Geometry: final body of the model. Coordinates: model frame, mm. Round coordinates to 2 decimals unless told otherwise and drop trailing zeros. Loops run counter-clockwise (first coordinate to the right, second up) from the corner with the lowest first, then second, coordinate; pieces in that order, holes last. Notation, with made-up numbers: (-17.5, -32.5) - (11.5, -32.5) arc R25 ccw to (11.5, -17.5) - close; hole circle Ø9 at (-40, -2.75). An arc over 180 degrees is marked (long way). Answer as a JSON object with one key per item and string values. Group by question number.
Item 1: Line query: line 1 (Y direction, x = 10.75, z = 183); line 2 (X direction, y = 27.25, z = 531.5); line 3 (X direction, y = 22.25, z = 193). Output: solid intervals per line, ascending.
Item 2: Section A-A (z = 459). Return the cut outline in (x, y).
Item 3: Section B-B (y = 22). Return the cut outline in (x, z).
Item 4: First-contact query: pin 1 (10 mm diameter, centred on x = 12, z = 390, fed in from +Y); pin 2 (3 mm diameter, centred on y = 6.5, z = 320, fed in from -X); pin 3 (1.5 mm diameter, centred on x = -2, z = 293.5, fed in from +Y). Flat tips, straight axial feed; report the tip coordinate or a pass-through.
```python
from build123d import *

# Parameters (mm, degrees)
BOSS_EXTRUDE1_DEPTH = 600


with BuildPart() as part:
    # Sketch1 → Boss-Extrude1 (new body)
    with BuildSketch(Plane.XY):
        with BuildLine():
            Line((15, 0), (-15, 0))
            Line((-15, 0), (-15, 4.7625))
            Line((-15, 4.7625), (-6, 4.7625))
            Line((-6, 4.7625), (-6, 11.1125))
            Line((-6, 11.1125), (-2.783018763, 16.684474949))
            ThreePointArc((-2.783018763, 16.684474949), (0, 28), (2.783018763, 16.684474949))
            Line((2.783018763, 16.684474949), (6, 11.1125))
            Line((6, 11.1125), (6, 4.7625))
            Line((6, 4.7625), (15, 4.7625))
            Line((15, 4.7625), (15, 0))
        make_face()
    extrude(amount=BOSS_EXTRUDE1_DEPTH)


solid = part.part
```
Values:
{
 "1": {"line 1": "y = 0 to 4.76", "line 2": "x = -2.9 to 2.9", "line 3": "x = -5.99 to 5.99"},
 "2": {"outline": "(-15, 0) - (15, 0) - (15, 4.76) - (6, 4.76) - (6, 11.11) - (2.78, 16.68) arc R6 ccw (long way) to (-2.78, 16.68) - (-6, 11.11) - (-6, 4.76) - (-15, 4.76) - close"},
 "3": {"outline": "(-6, 0) - (6, 0) - (6, 600) - (-6, 600) - close"},
 "4": {"pin 1": "stops at y = 4.76", "pin 2": "stops at x = -6", "pin 3": "stops at y = 27.87"}
}
